from build123d import *

# Parameters (mm, degrees)
SKETCH1_R             = 163.5
SKETCH1_R_2           = 158.7
BOSS_EXTRUDE1_DEPTH   = 767.5
BOSS_EXTRUDE2_START   = -10
SKETCH2_R             = 158.7
BOSS_EXTRUDE2_DEPTH   = 5
CHAMFER1_SIZE         = 0.5
M6_TAPPED_HOLE1_D     = 5
M6_TAPPED_HOLE1_DEPTH = 15
M6_TAPPED_HOLE1_TIP   = 1.502151548
SKETCH8_R             = 7
BOSS_EXTRUDE3_DEPTH   = 30
CHAMFER2_SIZE         = 0.5


with BuildPart() as part:
    # Sketch1 → Boss-Extrude1 (new, symmetric)
    with BuildSketch(Plane.XY):
        Circle(SKETCH1_R)
        Circle(SKETCH1_R_2, mode=Mode.SUBTRACT)
    extrude(amount=BOSS_EXTRUDE1_DEPTH, both=True)

    # Sketch2 → Boss-Extrude2 (add)
    with BuildSketch(Plane.XY.offset(767.5).offset(BOSS_EXTRUDE2_START)):
        Circle(SKETCH2_R)
    boss_extrude2 = extrude(amount=BOSS_EXTRUDE2_DEPTH)

    # Sketch5 → Revolve1 (revolve)
    with BuildSketch(Plane(origin=(0, 0, 0), x_dir=(0, 0, -1), z_dir=(1, 0, 0)), mode=Mode.PRIVATE) as revolve1_sk:
        Polygon((-779.5, 12), (779.5, 12), (779.5, 10.5), (810.5, 10.5), (810.5, 0), (-810.5, 0), (-810.5, 10.5), (-779.5, 10.5), align=None)
    revolve(revolve1_sk.sketch.rotate(Axis((0, 0, -810.5), (0, 0, -1)), 180), axis=Axis((0, 0, -810.5), (0, 0, -1)))

    # Chamfer1
    chamfer1_edges = [part.edges().sort_by_distance(p)[0] for p in [
        (0, 12, -779.5),
        (0, 12, 779.5),
        (0, 10.5, -810.5),
        (0, 10.5, 810.5),
    ]]
    chamfer(chamfer1_edges, length=CHAMFER1_SIZE)

    # M6 Tapped Hole1
    with Locations(Plane.XY.offset(810.5)):
        with Locations((0, 0)):
            Hole(M6_TAPPED_HOLE1_D / 2, depth=M6_TAPPED_HOLE1_DEPTH)
            with Locations((0, 0, -(M6_TAPPED_HOLE1_DEPTH + M6_TAPPED_HOLE1_TIP / 2))):  # 118° drill point
                Cone(0, M6_TAPPED_HOLE1_D / 2, M6_TAPPED_HOLE1_TIP, mode=Mode.SUBTRACT)

    # Mirror3: Boss-Extrude2 across plane
    add(boss_extrude2.mirror(Plane.XY))

    # Sketch8 → Boss-Extrude3 (add)
    with BuildSketch(Plane(origin=(0, 0, -810.5), x_dir=(-1, 0, 0), z_dir=(0, 0, -1))):
        with Locations(Location((0, 0, 0), (0, 0, 90))):
            Circle(SKETCH8_R)
    extrude(amount=BOSS_EXTRUDE3_DEPTH)

    # Chamfer2
    chamfer2_edges = [part.edges().sort_by_distance(p)[0] for p in [
        (0, -7, -840.5),
    ]]
    chamfer(chamfer2_edges, length=CHAMFER2_SIZE)


solid = part.part
Geometry: final body of the model. Coordinates: model frame, mm. A direction names the side the tool comes from. Coordinates: 2 decimals unless noted, no trailing zeros. Order: outer loops, then holes, each group sorted by start corner. A loop starts at its lowest first (then second) coordinate and runs counter-clockwise, first axis right, second up.
(1) First-contact query: pin 1 (12 mm diameter, centred on x = -71.5, z = -159, fed in from +Y); pin 2 (6 mm diameter, centred on x = 30.5, y = -49, fed in from +Z); pin 3 (8 mm diameter, centred on x = -30, z = 585, fed in from +Y). Flat tips, straight axial feed; report the tip coordinate or a pass-through.
(2) Section query C-C (y = -141). Return the cut outline in (x, z).
(3) Access query for faces 1 (the face through (-2, -33, -762.5)), 2 (the face through (-20.66, 157.35, 764.96)), 3 (the face through (-20.66, 157.35, -10.61)). Directions: +Z, -Z, +X, -X, +Y, -Y. A direction counts if a zero-diameter tool reaches every point of the face in a straight line with its end or side. Return the directions, or none.
(4) Material intervals for probe 1 along X at (y, z) = (-1.5, 446); probe 2 along Z at (x, y) = (92, 60); probe 3 along X at (y, z) = (0, 801.5), sorted ascending.
(5) Section query A-A (z = -437.5). Return the cut outline in (x, y), plus the area to 3 significant figures.
(6) Draft query along X for faces 4 (the face through (-35.444, -159.612, 10.745)), 5 (the face through (-2, -33, -757.5)), 6 (the face through (-86, 134, 767.5)). Return one class per face: pulls with the +X half, pulls with the -X half, needs draft (parallel to the pull), parting line crosses it, or undercut.
(7) Section query B-B (x = -77.5). Return the cut outline in (y, z).
Solution:
1. pin 1: stops at y = 149.81
1. pin 2: stops at z = 762.5
1. pin 3: stops at y = 161.42
2. outline: (-82.77, -767.5) - (-72.83, -767.5) - (-72.83, -762.5) - (72.83, -762.5) - (72.83, -767.5) - (82.77, -767.5) - (82.77, 767.5) - (72.83, 767.5) - (72.83, 762.5) - (-72.83, 762.5) - (-72.83, 767.5) - (-82.77, 767.5) - close; hole (-72.83, -757.5) - (72.83, -757.5) - (72.83, 757.5) - (-72.83, 757.5) - close
3. face 1: -Z
3. face 2: +Z
3. face 3: none
4. probe 1: x = -163.49 to -158.69, -11.91 to 11.91, 158.69 to 163.49
4. probe 2: z = -762.5 to -757.5, 757.5 to 762.5
4. probe 3: x = -10.5 to -2.5, 2.5 to 10.5
5. outline: circle Ø327 at (0, 0); circle Ø24 at (0, 0); hole circle Ø317.4 at (0, 0)
5. area: 5,310 mm2
6. face 4: parting line crosses it
6. face 5: undercut
6. face 6: needs draft
7. outline: (-143.97, -767.5) - (-138.49, -767.5) - (-138.49, -762.5) - (138.49, -762.5) - (138.49, -767.5) - (143.97, -767.5) - (143.97, 767.5) - (138.49, 767.5) - (138.49, 762.5) - (-138.49, 762.5) - (-138.49, 767.5) - (-143.97, 767.5) - close; hole (-138.49, -757.5) - (138.49, -757.5) - (138.49, 757.5) - (-138.49, 757.5) - close
